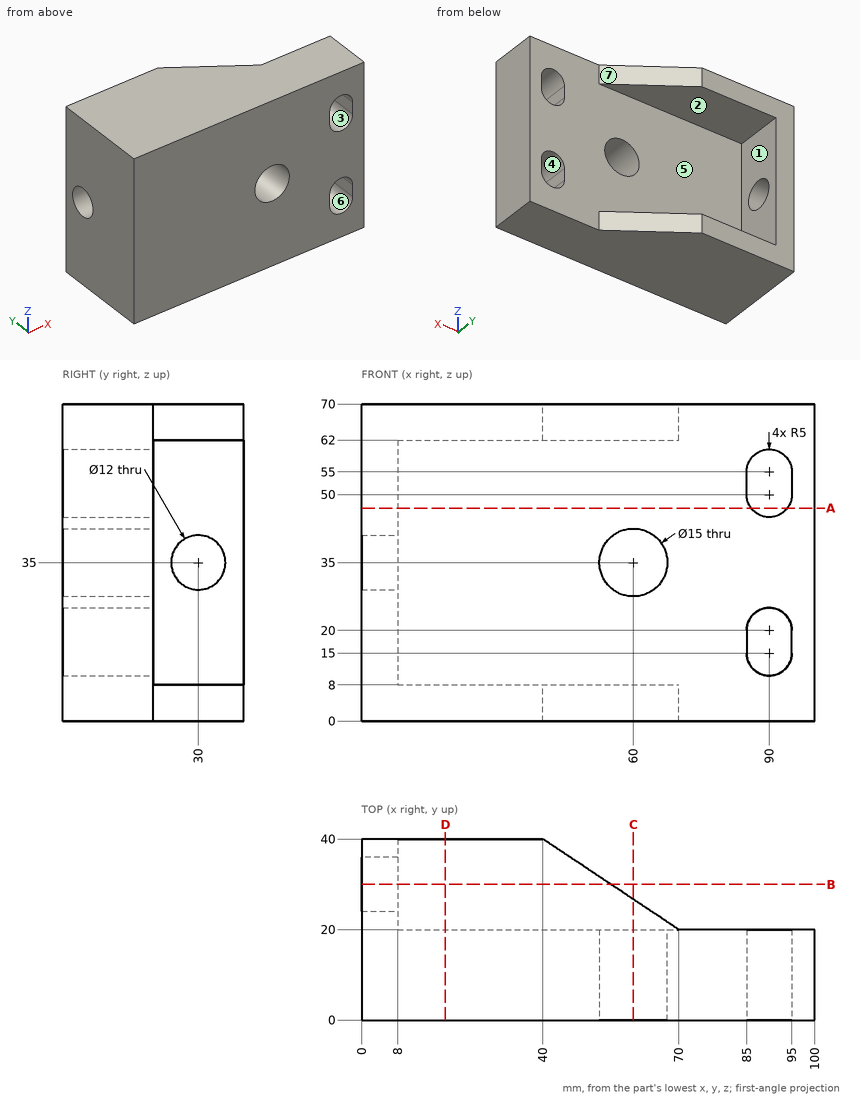
Print and shaded views of the part. All mm, measured from the part's lowest x, y and z. A direction names the side the tool comes from. Round coordinates to 2 decimals unless told otherwise and drop trailing zeros. Order: outer loops, then holes, each group sorted by start corner. A loop starts at its lowest first (then second) coordinate and runs counter-clockwise, first axis right, second up. Notation, with made-up numbers: (-29.5, 35.5) - (25.5, 35.5) arc R23 cw to (25.5, 58.5) - close; hole circle Ø1 at (59.25, -39). An arc over 180 degrees is marked (long way). Use a Markdown table: item, result.
1) Saw through at D-D on x = 18.5. Write the cut outline in (y, z).
Recorded:
| item | result |
|---|---|
| outline | (0, 0) - (40, 0) - (40, 8) - (20, 8) - (20, 62) - (40, 62) - (40, 70) - (0, 70) - close |
2) Saw through at A-A on z = 47. Write the cut outline in (x, y), and give its area (3 significant figures).
Recorded:
| item | result |
|---|---|
| outline | (0, 0) - (86, 0) - (86, 20) - (8, 20) - (8, 40) - (0, 40) - close; (94, 0) - (100, 0) - (100, 20) - (94, 20) - close |
| area | 2,000 mm² |
3) Tool access for the marked faces 5, 6 and 7: list every direction of +Z, -Z, +X, -X, +Y, -Y with a clear straight run to the whole face (end or side of a thin tool).
Recorded:
| item | result |
|---|---|
| face 5 | +X, +Y |
| face 6 | +Y, -Y |
| face 7 | +Z, -Z, +X, +Y |
4) Wall check: L1, parallel to Z at x = 62, y = 25; L2, parallel to Z at x = 4, y = 30; L3, parallel to X at y = 15.5, z = 23.5. Give the ranges that are in metal, low to high.
Recorded:
| item | result |
|---|---|
| L1 | z = 0 to 8, 62 to 70 |
| L2 | z = 0 to 29, 41 to 70 |
| L3 | x = 0 to 86.43, 93.57 to 100 |
5) Saw through at C-C on x = 60. Write the cut outline in (y, z), and give its area (3 significant figures).
Recorded:
| item | result |
|---|---|
| outline | (0, 0) - (26.67, 0) - (26.67, 8) - (20, 8) - (20, 27.5) - (0, 27.5) - close; (0, 42.5) - (20, 42.5) - (20, 62) - (26.67, 62) - (26.67, 70) - (0, 70) - close |
| area | 1,210 mm² |
6) Saw through at B-B on y = 30. Write the cut outline in (x, z), and give its area (3 significant figures).
Recorded:
| item | result |
|---|---|
| outline | (0, 0) - (55, 0) - (55, 8) - (8, 8) - (8, 29) - (0, 29) - close; (0, 41) - (8, 41) - (8, 62) - (55, 62) - (55, 70) - (0, 70) - close |
| area | 1,220 mm² |
7) Flat gauge pins, fed straight in: pin 1 Ø6 at (y, z) = (32.5, 26) entering from +X; pin 2 Ø6 at (x, z) = (72.5, 40.5) entering from +Y. Where does each tip first touch, or does it go through?
Recorded:
| item | result |
|---|---|
| pin 1 | stops at x = 8 |
| pin 2 | stops at y = 20 |
8) Pull direction X, two halves, no side cores. Call the marked faces 1, 2, 3 and 4: pulls with the +X half, pulls with the -X half, needs draft (parallel to the pull), parting line crosses it, or undercut.
Recorded:
| item | result |
|---|---|
| face 1 | pulls with the +X half |
| face 2 | needs draft |
| face 3 | undercut |
| face 4 | undercut |
